Verification items for the finished model (mm, model axes). Face numbers are marked on the shaded views. A direction names the side the tool comes from. Give positions to 0.01 mm unless a question says otherwise; leave off trailing zeros. Write each loop counter-clockwise with the first axis right and the second up, starting at its lowest first coordinate (ties: lowest second). Pieces come first, ordered by that corner, then holes. Notation, with made-up numbers: (14, 57) -> (25, 57) arc R26 cw to (25, 92) -> close; hole circle Ø2 at (64.5, 86). An arc over 180 degrees is marked (long way). Write item = value, one per line.
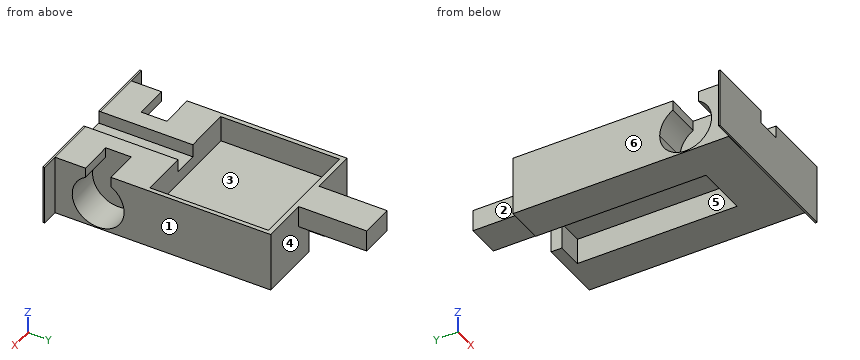
from build123d import *

# Parameters (mm, degrees)
F0_W      = 75
F0_H      = 35
F1_DEPTH  = 127
F3_DEPTH  = 20
F5_W      = 19.9898
F5_H      = 12.7
F6_DEPTH  = 40
F7_W      = 69.85
F7_H      = 69.85
F8_DEPTH  = 15.24
F9_W      = 95.2556729317
F9_H      = 34.9658876657
F10_DEPTH = 1
F11_W     = 14.6372080781
F11_H     = 57.15
F12_DEPTH = 7.62
F13_W     = 30.48
F13_H     = 93.98
F14_DEPTH = 15.24
F15_W     = 15.2369
F15_H     = 6.35
F16_DEPTH = 15.24


# Not quite as in the source:
# - a feature names something its author has since deleted; it is built from what else it names


with BuildPart() as f1:
    # F0 (on Front) → F1 (new body)
    with BuildSketch(Plane.XZ):
        Rectangle(F0_W, F0_H)
    extrude(amount=-F1_DEPTH)

    # F2 (on face) → F3 (cut)
    with BuildSketch(Plane.YZ.offset(37.5)):
        with BuildLine():
            ThreePointArc((17.9, 11.676062799), (25.4, 13.6444626123), (32.9, 11.676062799))
            Line((32.9, 11.676062799), (32.9, 17.5))
            Line((32.9, 17.5), (17.9, 17.5))
            Line((17.9, 17.5), (17.9, 11.676062799))
        make_face()
        with BuildLine():
            Line((32.9, 9.7889252245), (32.9, 11.676062799))
            ThreePointArc((32.9, 11.676062799), (25.4, 13.6444626123), (17.9, 11.676062799))
            Line((17.9, 11.676062799), (17.9, 9.7889252245))
            Line((17.9, 9.7889252245), (32.9, 9.7889252245))
        make_face()
        with BuildLine():
            ThreePointArc((17.9, 11.676062799), (17.6959593413, -14.8149434406), (40.672455682, -1.6279930697))
            ThreePointArc((40.672455682, -1.6279930697), (38.586950371, 6.076047589), (32.9, 11.676062799))
            Line((32.9, 11.676062799), (32.9, 9.7889252245))
            Line((32.9, 9.7889252245), (17.9, 9.7889252245))
            Line((17.9, 9.7889252245), (17.9, 11.676062799))
        make_face()
    extrude(amount=-F3_DEPTH, mode=Mode.SUBTRACT)

    # F4: F1 across plane


with BuildPart() as f1_1:
    add(f1.part)
    add(f1.part.mirror(Plane.YZ), mode=Mode.INTERSECT)

    # F5 (on face) → F6 (join)
    with BuildSketch(Plane(origin=(0, 127, 0), x_dir=(-1, 0, 0), z_dir=(0, 1, 0))):
        with Locations((0.0051, 11.15)):
            Rectangle(F5_W, F5_H)
    extrude(amount=F6_DEPTH)

    # F7 (on face) → F8 (cut)
    with BuildSketch(Plane.XY.offset(17.5)):
        with Locations((0.075, 89.2494911432)):
            Rectangle(F7_W, F7_H)
    extrude(amount=-F8_DEPTH, mode=Mode.SUBTRACT)

    # F9 (on Front) → F10 (join)
    with BuildSketch(Plane.XZ):
        Rectangle(F9_W, F9_H)
    extrude(amount=F10_DEPTH)

    # F11 (on face) → F12 (cut)
    with BuildSketch(Plane.XY.offset(17.5)):
        with Locations((0.0553701539, 27.575)):
            Rectangle(F11_W, F11_H)
    extrude(amount=-F12_DEPTH, mode=Mode.SUBTRACT)

    # F13 (on face) → F14 (cut)
    with BuildSketch(Plane(origin=(0, 0, -17.5), x_dir=(1, 0, 0), z_dir=(0, 0, -1))):
        with Locations((0.0031, -73.66)):
            Rectangle(F13_W, F13_H)
    extrude(amount=-F14_DEPTH, mode=Mode.SUBTRACT)

    # F15 (on face) → F16 (cut)
    with BuildSketch(Plane(origin=(0, 0, -17.5), x_dir=(1, 0, 0), z_dir=(0, 0, -1))):
        with Locations((-7.61845, -123.825)):
            Rectangle(F15_W, F15_H)
    extrude(amount=-F16_DEPTH, mode=Mode.SUBTRACT)


solid = f1_1.part
Item 1: Material ranges on line 1 (X direction, y = 108, z = 8); line 2 (X direction, y = 103, z = -4); line 3 (Y direction, x = -14.5, z = 11), recorded low to high.
Response values:
line_1 = -37.5 to -34.85, 35 to 37.5
line_2 = -37.5 to -15.24, 15.24 to 37.5
line_3 = -1 to 54.32, 124.17 to 127
Item 2: Sectioned sample at B-B on y = 99. Record the cut outline in (x, z).
Response values:
outline = (-37.5, -17.5) -> (-15.24, -17.5) -> (-15.24, -2.26) -> (15.24, -2.26) -> (15.24, -17.5) -> (37.5, -17.5) -> (37.5, 17.5) -> (35, 17.5) -> (35, 2.26) -> (-34.85, 2.26) -> (-34.85, 17.5) -> (-37.5, 17.5) -> close
Item 3: Go/stop test with flat-tipped pins: P1, Ø10, axis at x = 36, z = 10, coming from the +Y side; P2, Ø4, axis at x = 12.5, y = 86, coming from the +Z side; P3, Ø2, axis at y = 33, z = 8, coming from the -X side. Record where each tip stops, or that it passes through.
Response values:
P1 = 127
P2 = 2.26
P3 = -17.5
Item 4: Mould release check, pull along X, two halves, no side actions. Record for the marked faces 4, 5 and 6: +X half, -X half, draft (parallel to the pull), parting line (faces both ways), or undercut.
Response values:
face_4 = draft
face_5 = undercut
face_6 = -X half
Item 5: Sectioned sample at D-D on x = -40.5. Record the cut outline in (y, z).
Response values:
outline = (-1, -17.48) -> (0, -17.48) -> (0, 17.48) -> (-1, 17.48) -> close
Item 6: Sectioned sample at C-C on z = -9. Record the cut outline in (x, y).
Response values:
outline = (-47.63, -1) -> (47.63, -1) -> (47.63, 0) -> (37.5, 0) -> (37.5, 12.02) -> (17.5, 12.02) -> (17.5, 38.78) -> (37.5, 38.78) -> (37.5, 127) -> (0, 127) -> (0, 120.65) -> (15.24, 120.65) -> (15.24, 26.67) -> (-15.24, 26.67) -> (-15.24, 127) -> (-37.5, 127) -> (-37.5, 38.78) -> (-17.5, 38.78) -> (-17.5, 12.02) -> (-37.5, 12.02) -> (-37.5, 0) -> (-47.63, 0) -> close
Item 7: Set-up check for the marked faces 1, 2 and 3: record each of +Z, -Z, +X, -X, +Y, -Y from which the full face is reachable in a straight line by a thin tool's end or side.
Response values:
face_1 = +Z, -Z, +X, +Y
face_2 = +Z, -Z, -X, +Y
face_3 = +Z
